Geometry: final body of the model. Coordinates: model frame, mm. A direction names the side the tool comes from. Give positions to 0.01 mm unless a question says otherwise; leave off trailing zeros. Write each loop counter-clockwise with the first axis right and the second up, starting at its lowest first coordinate (ties: lowest second). Pieces come first, ordered by that corner, then holes.
```python
from build123d import *

# Parameters (mm, degrees)
SKETCH1_W            = 80
SKETCH1_H            = 50
SKETCH1_R            = 1.75
BOSS_EXTRUDE1_DEPTH  = 1.6
SKETCH2_W            = 4.2
SKETCH2_H            = 9.5
SKETCH2_W_2          = 7.67
SKETCH2_H_2          = 10.56
BOSS_EXTRUDE2_DEPTH  = 10.5
CHAMFER1_SIZE        = 2
CHAMFER2_SIZE        = 1
SKETCH3_R            = 1.25
BOSS_EXTRUDE3_DEPTH  = 1.5
CUT_EXTRUDE1_START   = -0.5
CUT_EXTRUDE1_DEPTH   = 0.5
SKETCH5_W            = 33.5
SKETCH5_H            = 17
BOSS_EXTRUDE4_DEPTH  = 4.5
BOSS_EXTRUDE5_DEPTH  = 2.5
SKETCH7_W            = 6
SKETCH7_H            = 6
BOSS_EXTRUDE6_DEPTH  = 3.5
SKETCH8_R            = 1.5
BOSS_EXTRUDE7_DEPTH  = 6.5
SKETCH9_W            = 36
SKETCH9_H            = 25
BOSS_EXTRUDE8_DEPTH  = 1.5
SKETCH10_W           = 36
SKETCH10_H           = 1.5
SKETCH10_H_2         = 1
BOSS_EXTRUDE9_DEPTH  = 3.5
SKETCH11_R           = 5
BOSS_EXTRUDE10_DEPTH = 13.5
SKETCH12_R           = 10.25
SKETCH12_R_2         = 6.25
BOSS_EXTRUDE11_DEPTH = 8.25


with BuildPart() as part:
    # Sketch1 → Boss-Extrude1 (new body)
    with BuildSketch(Plane.XY):
        Rectangle(SKETCH1_W, SKETCH1_H)
        with Locations((-37.5, 22.5)):
            Circle(SKETCH1_R, mode=Mode.SUBTRACT)
        with Locations((-37.5, -22.5)):
            Circle(SKETCH1_R, mode=Mode.SUBTRACT)
        with Locations((37.5, -22.5)):
            Circle(SKETCH1_R, mode=Mode.SUBTRACT)
        with Locations((37.5, 22.5)):
            Circle(SKETCH1_R, mode=Mode.SUBTRACT)
    extrude(amount=BOSS_EXTRUDE1_DEPTH)

    # Sketch2 → Boss-Extrude2 (add)
    with BuildSketch(Plane.XY.offset(1.6)):
        with Locations((24.7, -14.25)):
            Rectangle(SKETCH2_W, SKETCH2_H)
        with Locations((30.4, -14.25)):
            Rectangle(SKETCH2_W, SKETCH2_H)
        with Locations((36.165, 12.22)):
            Rectangle(SKETCH2_W_2, SKETCH2_H_2)
        with Locations((-36.165, 12.22)):
            Rectangle(SKETCH2_W_2, SKETCH2_H_2)
    extrude(amount=BOSS_EXTRUDE2_DEPTH)

    # Chamfer1
    chamfer1_edges = [part.edges().sort_by_distance(p)[0] for p in [
        (32.33, 12.22, 12.1),
        (-32.33, 12.22, 12.1),
    ]]
    chamfer(chamfer1_edges, length=CHAMFER1_SIZE)

    # Chamfer2
    chamfer2_edges = [part.edges().sort_by_distance(p)[0] for p in [
        (40, 12.22, 12.1),
        (-40, 12.22, 12.1),
    ]]
    chamfer(chamfer2_edges, length=CHAMFER2_SIZE)

    # Sketch3 → Boss-Extrude3 (add)
    with BuildSketch(Plane.XY.offset(12.1)):
        with Locations(Location((23.85, -17.75, 0), (0, 0, 180))):
            Circle(SKETCH3_R)
        with Locations(Location((29.55, -17.75, 0), (0, 0, 180))):
            Circle(SKETCH3_R)
    extrude(amount=BOSS_EXTRUDE3_DEPTH)

    # Sketch4 → Cut-Extrude1 (cut)
    with BuildSketch(Plane.XY.offset(13.6).offset(CUT_EXTRUDE1_START)):
        with BuildLine():
            Line((23.6, -16.525255129), (23.6, -18.974744871))
            ThreePointArc((23.6, -18.974744871), (23.85, -19), (24.1, -18.974744871))
            Line((24.1, -18.974744871), (24.1, -16.525255129))
            ThreePointArc((24.1, -16.525255129), (23.85, -16.5), (23.6, -16.525255129))
        make_face()
        with BuildLine():
            Line((28.991531245, -18.868307941), (29.625505842, -16.502282537))
            ThreePointArc((29.625505842, -16.502282537), (29.873523806, -16.542592717), (30.108468755, -16.631692059))
            Line((30.108468755, -16.631692059), (29.474494158, -18.997717463))
            ThreePointArc((29.474494158, -18.997717463), (29.226476194, -18.957407283), (28.991531245, -18.868307941))
        make_face()
    extrude(amount=CUT_EXTRUDE1_DEPTH, mode=Mode.SUBTRACT)

    # Sketch5 → Boss-Extrude4 (add)
    with BuildSketch(Plane.XY.offset(1.6)):
        with Locations((-2.25, -12)):
            Rectangle(SKETCH5_W, SKETCH5_H)
    extrude(amount=BOSS_EXTRUDE4_DEPTH)

    # Sketch6 → Boss-Extrude5 (add)
    with BuildSketch(Plane.XY.offset(1.6)):
        Polygon((-24, -18.25), (-19, -20.25), (-19, -3.75), (-24, -5.75), align=None)
    extrude(amount=BOSS_EXTRUDE5_DEPTH)

    # Sketch7 → Boss-Extrude6 (add)
    with BuildSketch(Plane.XY.offset(1.6)):
        with Locations((-31, -16.5)):
            Rectangle(SKETCH7_W, SKETCH7_H)
        with Locations((-31, -6)):
            Rectangle(SKETCH7_W, SKETCH7_H)
    extrude(amount=BOSS_EXTRUDE6_DEPTH)

    # Sketch8 → Boss-Extrude7 (add)
    with BuildSketch(Plane.XY.offset(5.1)):
        with Locations(Location((-31, -6, 0), (0, 0, 180))):
            Circle(SKETCH8_R)
        with Locations(Location((-31, -16.5, 0), (0, 0, 180))):
            Circle(SKETCH8_R)
    extrude(amount=BOSS_EXTRUDE7_DEPTH)

    # Sketch9 → Boss-Extrude8 (add)
    with BuildSketch(Plane.XY.offset(1.6)):
        with Locations((-2.25, 12.5)):
            Rectangle(SKETCH9_W, SKETCH9_H)
    extrude(amount=BOSS_EXTRUDE8_DEPTH)

    # Sketch10 → Boss-Extrude9 (add)
    with BuildSketch(Plane.XY.offset(3.1)):
        with Locations((-2.25, 0.75)):
            Rectangle(SKETCH10_W, SKETCH10_H)
        with Locations((-2.25, 24.25)):
            Rectangle(SKETCH10_W, SKETCH10_H)
        with Locations((-2.25, 3.993100162)):
            Rectangle(SKETCH10_W, SKETCH10_H_2)
        with Locations((-2.25, 6.986200324)):
            Rectangle(SKETCH10_W, SKETCH10_H_2)
        with Locations((-2.25, 9.979300486)):
            Rectangle(SKETCH10_W, SKETCH10_H_2)
        with Locations((-2.25, 12.972400648)):
            Rectangle(SKETCH10_W, SKETCH10_H_2)
        with Locations((-2.25, 15.96550081)):
            Rectangle(SKETCH10_W, SKETCH10_H_2)
        with Locations((-2.25, 19.982750405)):
            Rectangle(SKETCH10_W, SKETCH10_H_2)
    extrude(amount=BOSS_EXTRUDE9_DEPTH)

    # Sketch11 → Boss-Extrude10 (add)
    with BuildSketch(Plane(origin=(0, 0, 0), x_dir=(-1, 0, 0), z_dir=(0, 0, -1))):
        with Locations(Location((-26, 20, 0), (0, 0, 90))):
            Circle(SKETCH11_R)
        with Locations(Location((25, 14, 0), (0, 0, 180))):
            Circle(SKETCH11_R)
    extrude(amount=BOSS_EXTRUDE10_DEPTH)

    # Sketch12 → Boss-Extrude11 (add)
    with BuildSketch(Plane(origin=(0, 0, 0), x_dir=(-1, 0, 0), z_dir=(0, 0, -1))):
        with Locations(Location((-20.5, 4, 0), (0, 0, 180))):
            Circle(SKETCH12_R)
        with Locations((-20.5, 4)):
            Circle(SKETCH12_R_2, mode=Mode.SUBTRACT)
    extrude(amount=BOSS_EXTRUDE11_DEPTH)


solid = part.part
```
Item 1: Pull-direction query (X, two-part tool) for faces 6 (the face through (-2, -12, 6.1)), 7 (the face through (30, -9.5, 7)); classes: +X half, -X half, draft (parallel to the pull), parting line (faces both ways), or undercut.
Found:
face 6: undercut
face 7: draft
Item 2: Line query: L1, parallel to Y at x = 37.5, z = 0.75; L2, parallel to Z at x = 25, y = -8; L3, parallel to Z at x = 11, y = -13.5. Output: solid intervals per line, ascending.
Found:
L1: y = -25 to -24.25, -20.75 to 20.75, 24.25 to 25
L2: z = 0 to 1.6
L3: z = 0 to 6.1
Item 3: Pin query (flat end, axial travel): pin 1 Ø10 at (x, y) = (6.5, 17.5) entering from +Z; pin 2 Ø0.6 at (x, y) = (-3.5, 14.5) entering from +Z; pin 3 Ø6 at (x, z) = (-37.5, 8) entering from +Y; pin 4 Ø6 at (x, z) = (2.5, -1) entering from +Y. Return the tip coordinate at first contact, or that it passes through.
Found:
pin 1: stops at z = 6.6
pin 2: stops at z = 3.1
pin 3: stops at y = 17.5
pin 4: stops at y = 25
Item 4: Section A-A, the plane z = -3.25. Return the cut outline in (x, y), plus the area to 3 significant figures.
Found:
outline: circle Ø10 at (-25, 14); circle Ø20.5 at (20.5, 4); circle Ø10 at (26, 20); hole circle Ø12.5 at (20.5, 4)
area: 364 mm2
Item 5: Reachability of faces 1 (the face through (-3, 4.493, 5)), 2 (the face through (-32.4, -4.6, 5.1)), 3 (the face through (-31, -13.5, 3)), 4 (the face through (21.12, 18.92, -6.66)), 5 (the face through (22.6, -14, 7)) from +Z, -Z, +X, -X, +Y, -Y: full face, straight path, thin tool, end or side. Return the list, or none.
Found:
face 1: +Z, +X, -X
face 2: +Z
face 3: +Z, -X
face 4: -Z
face 5: +Z, +Y, -Y
Item 6: Section B-B, the plane x = -25. Return the cut outline in (y, z).
Found:
outline: (-25, 0) - (9, 0) - (9, -13.5) - (19, -13.5) - (19, 0) - (25, 0) - (25, 1.6) - (-25, 1.6) - close
